```python
from build123d import *

# Parameters (mm, degrees)
SKETCH1_W                      = 56.2
SKETCH1_H                      = 30
BOSS_EXTRUDE1_DEPTH            = 5
SKETCH3_W                      = 56.2
SKETCH3_H                      = 30
BOSS_EXTRUDE2_DEPTH            = 3
SKETCH4_R                      = 1.7
CUT_EXTRUDE2_DEPTH             = 8
BOSS_EXTRUDE3_DEPTH            = 12
BOSS_EXTRUDE4_DEPTH            = 10
BOSS_EXTRUDE4_DEPTH_BACK       = 10
CUT_EXTRUDE3_REACH             = 38.4
CUT_EXTRUDE3_DIRECTION_2_REACH = 38.4
SKETCH8_R                      = 2.6
CUT_EXTRUDE4_DEPTH             = 4


with BuildPart() as part:
    # Sketch1 → Boss-Extrude1 (new body)
    with BuildSketch(Plane.XY):
        with Locations((28.1, -15)):
            Rectangle(SKETCH1_W, SKETCH1_H)
    extrude(amount=BOSS_EXTRUDE1_DEPTH)

    # Sketch3 → Boss-Extrude2 (add)
    with BuildSketch(Plane.XY.offset(5)):
        with Locations((28.1, -15)):
            Rectangle(SKETCH3_W, SKETCH3_H)
    extrude(amount=BOSS_EXTRUDE2_DEPTH)

    # Sketch4 → Cut-Extrude2 (cut)
    with BuildSketch(Plane(origin=(0, 0, 0), x_dir=(-1, 0, 0), z_dir=(0, 0, -1))):
        with Locations((-49.2, -7)):
            Circle(SKETCH4_R)
        with Locations((-7, -7)):
            Circle(SKETCH4_R)
        with Locations((-7, -23)):
            Circle(SKETCH4_R)
        with Locations((-49.2, -23)):
            Circle(SKETCH4_R)
    extrude(amount=-CUT_EXTRUDE2_DEPTH, mode=Mode.SUBTRACT)

    # Sketch5 → Boss-Extrude3 (add)
    with BuildSketch(Plane(origin=(0, 0, 0), x_dir=(1, 0, 0), z_dir=(0, 1, 0))):
        with BuildLine():
            Line((44.5, 0), (11.7, 0))
            Line((11.7, 0), (11.7, 15))
            Line((11.7, 15), (-8.3, 15))
            Line((-8.3, 15), (-8.3, 65))
            ThreePointArc((-8.3, 65), (-6.835533906, 68.535533906), (-3.3, 70))
            Line((-3.3, 70), (59.5, 70))
            ThreePointArc((59.5, 70), (63.035533906, 68.535533906), (64.5, 65))
            Line((64.5, 65), (64.5, 15))
            Line((64.5, 15), (44.5, 15))
            Line((44.5, 15), (44.5, 0))
        make_face()
    extrude(amount=-BOSS_EXTRUDE3_DEPTH)

    # Sketch6 → Boss-Extrude4 (add, two sides)
    with BuildSketch(Plane(origin=(28.1, 0, 0), x_dir=(0, 0, -1), z_dir=(1, 0, 0))) as boss_extrude4_sk:
        Polygon((0, -12), (0, -30), (70, -12), align=None)
    extrude(amount=BOSS_EXTRUDE4_DEPTH)
    extrude(boss_extrude4_sk.sketch, amount=-BOSS_EXTRUDE4_DEPTH_BACK)

    # Sketch7 → Cut-Extrude3 (cut, up to next)
    with BuildSketch(Plane(origin=(28.1, 0, 0), x_dir=(0, 0, -1), z_dir=(1, 0, 0)), mode=Mode.PRIVATE) as cut_extrude3_sk1:
        Polygon((8, -12), (8, -22), (46.888888889, -12), align=None)
    cut_extrude3_tool1 = extrude(cut_extrude3_sk1.sketch, amount=-CUT_EXTRUDE3_REACH, mode=Mode.PRIVATE) & part.part
    add(cut_extrude3_tool1.solids().sort_by_distance((28.1, -15.333333, -20.962963))[0], mode=Mode.SUBTRACT)

    # Sketch7 → Cut-Extrude3 direction 2 (cut, up to next)
    with BuildSketch(Plane(origin=(28.1, 0, 0), x_dir=(0, 0, -1), z_dir=(1, 0, 0)), mode=Mode.PRIVATE) as cut_extrude3_direction_2_sk1:
        Polygon((8, -12), (8, -22), (46.888888889, -12), align=None)
    cut_extrude3_direction_2_tool1 = extrude(cut_extrude3_direction_2_sk1.sketch, amount=CUT_EXTRUDE3_DIRECTION_2_REACH, mode=Mode.PRIVATE) & part.part
    add(cut_extrude3_direction_2_tool1.solids().sort_by_distance((28.1, -15.333333, -20.962963))[0], mode=Mode.SUBTRACT)

    # Sketch8 → Cut-Extrude4 (cut)
    with BuildSketch(Plane(origin=(0, 0, 0), x_dir=(-1, 0, 0), z_dir=(0, 0, -1))):
        with Locations((-49.2, -7)):
            Circle(SKETCH8_R)
        with Locations((-7, -7)):
            Circle(SKETCH8_R)
        with Locations((-7, -23)):
            Circle(SKETCH8_R)
        with Locations((-49.2, -23)):
            Circle(SKETCH8_R)
    extrude(amount=-CUT_EXTRUDE4_DEPTH, mode=Mode.SUBTRACT)


solid = part.part
```
Model file for the job. Use its own axes, mm. A direction names the side the tool comes from. Give positions to 0.01 mm unless a question says otherwise; leave off trailing zeros. Loops run counter-clockwise (first coordinate to the right, second up) from the corner with the lowest first, then second, coordinate; pieces in that order, holes last. Notation, with made-up numbers: (69, 3) -> (124, 3) arc R32 cw to (124, 39) -> close; hole circle Ø8 at (11, 21.25). An arc over 180 degrees is marked (long way). Use CSV: the item, a comma, the result in double quotes. Start each with the question number.
1) Tool access for faces 4 (the flat face through (49, -9, 4)), 5 (the flat face through (2, -6, -15)), 6 (the flat face through (28.24, -17.07, -27.17)), 7 (the flat face through (55, -6, -15)): list every direction of +Z, -Z, +X, -X, +Y, -Y with a clear straight run to the whole face (end or side of a thin tool).
2) Slice it at B-B on y = -7. Give the number of separate pieces and of enclosed holes in the cut face, plus the area to 3 significant figures.
3) Slice it at C-C on z = -12. Give the cut face in (x, y).
4) Flat gauge pins, fed straight in: pin 1 Ø2 at (x, y) = (7, -7) entering from +Z; pin 2 Ø10 at (y, z) = (-23, -42) entering from -X; pin 3 Ø8 at (x, z) = (39.5, -18.5) entering from -Y; pin 4 Ø3 at (x, y) = (49.2, -23) entering from -Z. Where does each tip first touch, or does it go through?
5) Slice it at A-A on x = 49.2. Give the cut face in (y, z), plus the area to 3 significant figures.
6) Slice it at D-D on x = 25.5. Give the cut face in (y, z), plus the area to 3 significant figures.
7) Wall check: line 1 (Y direction, x = 7, z = 5.75); line 2 (Y direction, x = 7, z = 0.9); line 3 (Z direction, x = 1, y = -1.25). Give the ranges that are in metal, low to high.
8) Mould opens along Y. For faces 1 (the flat face through (56.2, -15, 4)), 2 (the flat face through (5, -8, 4)), 3 (the flat face through (28, -21, -35)) say: released by +Y, released by -Y, zero draft, split by the parting line, or undercut.
Computed values:
1,face 4,"none"
1,face 5,"-X, +Y, -Y"
1,face 6,"+X, -X"
1,face 7,"+X, +Y, -Y"
2,separate pieces,"3"
2,enclosed holes,"0"
2,area,"4,870 mm^2"
3,outline,"(11.7, -12) -> (44.5, -12) -> (44.5, 0) -> (11.7, 0) -> close; (18.1, -26.91) -> (38.1, -26.91) -> (38.1, -20.97) -> (18.1, -20.97) -> close"
4,pin 1,"stops at z = -15"
4,pin 2,"stops at x = 18.1"
4,pin 3,"stops at y = -26.21"
4,pin 4,"passes through"
5,outline,"(-30, 0) -> (-25.6, 0) -> (-25.6, 4) -> (-24.7, 4) -> (-24.7, 8) -> (-30, 8) -> close; (-21.3, 4) -> (-20.4, 4) -> (-20.4, 0) -> (-9.6, 0) -> (-9.6, 4) -> (-8.7, 4) -> (-8.7, 8) -> (-21.3, 8) -> close; (-12, -70) -> (0, -70) -> (0, -15) -> (-12, -15) -> close; (-5.3, 4) -> (-4.4, 4) -> (-4.4, 0) -> (0, 0) -> (0, 8) -> (-5.3, 8) -> close"
5,area,"831 mm^2"
6,outline,"(-30, 0) -> (-12, -70) -> (0, -70) -> (0, 8) -> (-30, 8) -> close; hole (-22, -8) -> (-12, -46.89) -> (-12, -8) -> close"
6,area,"1,520 mm^2"
7,line 1,"y = -30 to -24.7, -21.3 to -8.7, -5.3 to 0"
7,line 2,"y = -30 to -25.6, -20.4 to -9.6, -4.4 to 0"
7,line 3,"z = -70 to -15, 0 to 8"
8,face 1,"zero draft"
8,face 2,"undercut"
8,face 3,"released by -Y"
